Check sheet for the modelled part. Datum: model origin and axes. Units: mm. Face numbers are marked on the shaded views. A direction names the side the tool comes from. Round coordinates to 2 decimals unless told otherwise and drop trailing zeros. Loops run counter-clockwise (first coordinate to the right, second up) from the corner with the lowest first, then second, coordinate; pieces in that order, holes last. Notation, with made-up numbers: (12, -7) -> (41, -7) arc R14 cw to (41, 12) -> close; hole circle Ø7 at (41, -30). An arc over 180 degrees is marked (long way). One line per item, written item: value. Start each with the question number.
1. Cross-section at B-B on z = 0.5. Record the cut outline in (x, y).
2. Go/stop test with flat-tipped pins: pin 1 (11 mm diameter, centred on x = -2, y = 0.5, fed in from -Z); pin 2 (5 mm diameter, centred on x = 0, y = 5, fed in from -Z). Record where each tip stops, or that it passes through.
3. Cross-section at A-A on z = -1.75. Record the cut outline in (x, y).
4. Material ranges on L1, parallel to X at y = 5, z = 0.35; L2, parallel to Y at x = 0, z = -0.15; L3, parallel to X at y = -2, z = -3.25, recorded low to high.
5. Cross-section at C-C on y = -2. Record the cut outline in (x, z), then the cut area to 3 significant figures.
6. Cross-section at D-D on x = 0. Record the cut outline in (y, z).
7. Release check for a two-part mould opening along Y. For the marked faces 3, 4, 5 and 6 record: +Y half, -Y half, draft (parallel to the pull), parting line (faces both ways), or undercut.
8. Set-up check for the marked faces 1 and 2: record each of +Z, -Z, +X, -X, +Y, -Y from which the full face is reachable in a straight line by a thin tool's end or side.
from build123d import *

# Parameters (mm, degrees)
SKETCH3_W                                       = 20
SKETCH3_H                                       = 30
BOSS_EXTRUDE1_DEPTH                             = 4
SKETCH4_W                                       = 12
SKETCH4_H                                       = 30
CUT_EXTRUDE1_DEPTH                              = 3
CSK_FOR_M5_FLAT_HEAD_MACHINE_SCREW1_D           = 5.8
CSK_FOR_M5_FLAT_HEAD_MACHINE_SCREW1_CSINK_D     = 10.4
CSK_FOR_M5_FLAT_HEAD_MACHINE_SCREW1_CSINK_ANGLE = 90
BOSS_EXTRUDE2_DEPTH                             = 3
FILLET1_R                                       = 1


with BuildPart() as part:
    # Sketch3 → Boss-Extrude1 (new body, symmetric)
    with BuildSketch(Plane.XY):
        Rectangle(SKETCH3_W, SKETCH3_H)
    extrude(amount=BOSS_EXTRUDE1_DEPTH, both=True)

    # Sketch4 → Cut-Extrude1 (cut)
    with BuildSketch(Plane(origin=(0, 0, -4), x_dir=(-1, 0, 0), z_dir=(0, 0, -1))):
        Rectangle(SKETCH4_W, SKETCH4_H)
    extrude(amount=-CUT_EXTRUDE1_DEPTH, mode=Mode.SUBTRACT)

    # CSK for M5 Flat Head Machine Screw1 (through all)
    with Locations(Plane(origin=(0, 5, 4), x_dir=(1, 0, 0), z_dir=(0, 0, 1))):
        with Locations((0, 0)):
            CounterSinkHole(CSK_FOR_M5_FLAT_HEAD_MACHINE_SCREW1_D / 2, CSK_FOR_M5_FLAT_HEAD_MACHINE_SCREW1_CSINK_D / 2, counter_sink_angle=CSK_FOR_M5_FLAT_HEAD_MACHINE_SCREW1_CSINK_ANGLE)

    # Sketch7 → Boss-Extrude2 (add)
    with BuildSketch(Plane(origin=(0, 0, -1), x_dir=(-1, 0, 0), z_dir=(0, 0, -1))):
        with BuildLine():
            Line((5.462217277, 2.51722284), (-2.5, -15))
            Line((-2.5, -15), (6, -15))
            Line((6, -15), (6, 5))
            ThreePointArc((6, 5), (5.864013287, 3.729823567), (5.462217277, 2.51722284))
        make_face()
    extrude(amount=BOSS_EXTRUDE2_DEPTH)

    # Fillet1
    fillet1_edges = [part.edges().sort_by_distance(p)[0] for p in [
        (6, -15, -2.5),
        (6, 15, -2.5),
        (-6, 15, -2.5),
        (2.5, -15, -2.5),
        (-10, 15, 0),
        (10, 15, 0),
        (10, -15, 0),
        (-10, -15, 0),
    ]]
    fillet(fillet1_edges, radius=FILLET1_R)


solid = part.part
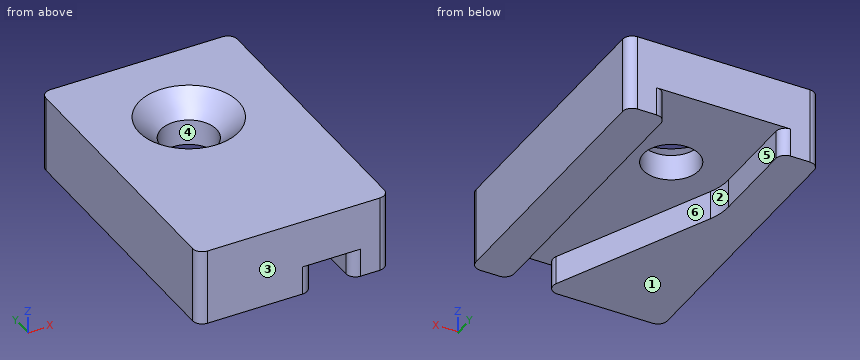
Taken from the geometry:
1. outline: (-10, -14) arc R1 ccw to (-9, -15) -> (9, -15) arc R1 ccw to (10, -14) -> (10, 14) arc R1 ccw to (9, 15) -> (-9, 15) arc R1 ccw to (-10, 14) -> close; hole circle Ø5.8 at (0, 5)
2. pin 1: stops at z = -4
2. pin 2: passes through
3. outline: (-10, -14) arc R1 ccw to (-9, -15) -> (0.95, -15) arc R1 ccw to (1.86, -13.59) -> (-5.46, 2.52) arc R6 cw to (-6, 5) -> (-6, 14) arc R1 ccw to (-7, 15) -> (-9, 15) arc R1 ccw to (-10, 14) -> close; (6, -14) arc R1 ccw to (7, -15) -> (9, -15) arc R1 ccw to (10, -14) -> (10, 14) arc R1 ccw to (9, 15) -> (7, 15) arc R1 ccw to (6, 14) -> close
4. L1: x = -10 to -2.9, 2.9 to 10
4. L2: y = -15 to 2.1, 7.9 to 15
4. L3: x = -10 to -3.41, 6 to 10
5. outline: (-10, -4) -> (-3.41, -4) -> (-3.41, -1) -> (6, -1) -> (6, -4) -> (10, -4) -> (10, 4) -> (-10, 4) -> close
5. area: 132 mm2
6. outline: (-15, -4) -> (-9.5, -4) -> (-9.5, -1) -> (2.1, -1) -> (2.1, 1.7) -> (-0.2, 4) -> (-15, 4) -> close; (7.9, -1) -> (15, -1) -> (15, 4) -> (10.2, 4) -> (7.9, 1.7) -> close
7. face 3: -Y half
7. face 4: undercut
7. face 5: draft
7. face 6: +Y half
8. face 1: -Z, +X, -X, +Y, -Y
8. face 2: -Z, +Y
